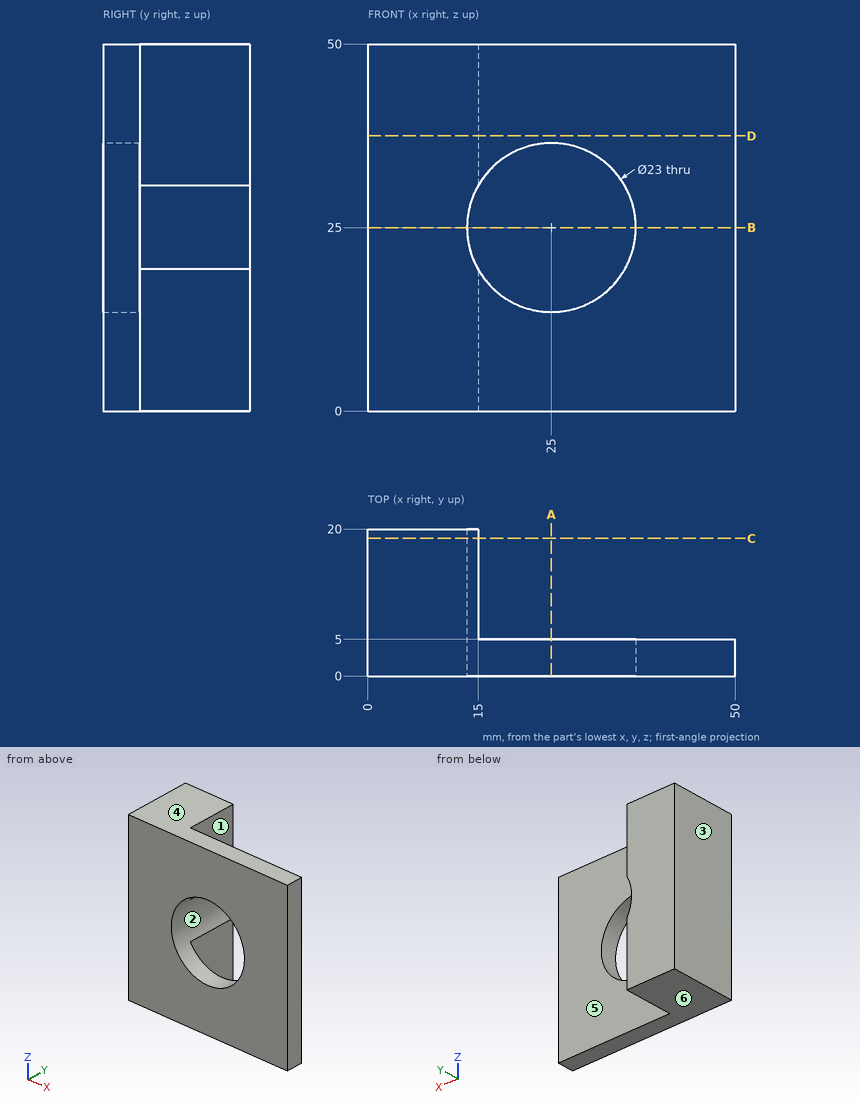
Check sheet for the drawn part. Datum: minimum x, y, z corner. Units: mm. A direction names the side the tool comes from. Round coordinates to 2 decimals unless told otherwise and drop trailing zeros. Order: outer loops, then holes, each group sorted by start corner. A loop starts at its lowest first (then second) coordinate and runs counter-clockwise, first axis right, second up. Notation, with made-up numbers: (88, -11.75) -> (97, -11.75) arc R12 ccw to (97, -7.75) -> close; hole circle Ø7 at (-11, -27). An arc over 180 degrees is marked (long way). Put each result on its own line as item: value.
1) Material ranges on line 1 (X direction, y = 4.5, z = 25); line 2 (X direction, y = 14, z = 25); line 3 (X direction, y = 17.5, z = 39.5), recorded low to high.
Final values:
line 1: x = 0 to 13.5, 36.5 to 50
line 2: x = 0 to 13.5
line 3: x = 0 to 15
2) Section check D-D (z = 37.5). Record the cut outline in (x, y), then the cut area to 3 significant figures.
Final values:
outline: (0, 0) -> (50, 0) -> (50, 5) -> (15, 5) -> (15, 20) -> (0, 20) -> close
area: 475 mm^2
3) Section check A-A (x = 25). Record the cut outline in (y, z).
Final values:
outline: (0, 0) -> (5, 0) -> (5, 13.5) -> (0, 13.5) -> close; (0, 36.5) -> (5, 36.5) -> (5, 50) -> (0, 50) -> close
4) Section check B-B (z = 25). Record the cut outline in (x, y), then the cut area to 4 significant figures.
Final values:
outline: (0, 0) -> (13.5, 0) -> (13.5, 20) -> (0, 20) -> close; (36.5, 0) -> (50, 0) -> (50, 5) -> (36.5, 5) -> close
area: 337.5 mm^2
5) Depth check by flat-ended pin: pin 1 (7.5 mm diameter, centred on y = 15.5, z = 12, fed in from +X); pin 2 (12 mm diameter, centred on x = 42.5, z = 26.5, fed in from +Y); pin 3 (8 mm diameter, centred on y = 6.5, z = 25.5, fed in from -X). Enter the tip coordinate at first touch or a pass-through.
Final values:
pin 1: stops at x = 15
pin 2: stops at y = 5
pin 3: stops at x = 0
6) Section check C-C (y = 18.75). Record the cut outline in (x, z).
Final values:
outline: (0, 0) -> (15, 0) -> (15, 19.32) arc R11.5 cw to (15, 30.68) -> (15, 50) -> (0, 50) -> close
7) Set-up check for the marked faces 5 and 6: record each of +Z, -Z, +X, -X, +Y, -Y from which the full face is reachable in a straight line by a thin tool's end or side.
Final values:
face 5: +Z, -Z, +X, +Y
face 6: -Z, +X, -X, +Y, -Y
8) Mould release check, pull along X, two halves, no side actions. Record for the marked faces 1, 2, 3 and 4: +X half, -X half, draft (parallel to the pull), parting line (faces both ways), or undercut.
Final values:
face 1: +X half
face 2: undercut
face 3: -X half
face 4: draft
